For this review, take the finished solid that the model builds, in its own axes (mm). A direction names the side the tool comes from. Coordinates: 2 decimals unless noted, no trailing zeros. Loops run counter-clockwise (first coordinate to the right, second up) from the corner with the lowest first, then second, coordinate; pieces in that order, holes last. Notation, with made-up numbers: (-4.75, 32) - (32.25, 32) arc R17 cw to (32.25, 41) - close; hole circle Ø4 at (59, -7). An arc over 180 degrees is marked (long way). Use one line per item in the form item = value. Start each with the question number.
1. Machinability: for faces 1 (the face through (21, -87, 2)), 2 (the face through (27.5, -95, 2)), 3 (the face through (52.25, -102, 2)), 4 (the face through (-65, -1, 2)), which of the approach directions +Z, -Z, +X, -X, +Y, -Y give a long, thin tool a straight path to every point of the face, cutting with its end or side? Answer none if there is none.
2. To check wall thickness, follow probe 1 along Y at (x, z) = (28, 4); probe 2 along Y at (x, z) = (20.5, 2.55); probe 3 along Y at (x, z) = (-25, 2.1). State the ranges of each line that lie inside material, in increasing order.
3. Draft analysis for pull direction Y (two halves, no side actions). For faces 5 (the face through (-59, -100, 2)), 6 (the face through (29, -86, 2)), 7 (the face through (-27.5, -79, 2)), state which applies: +Y half, -Y half, draft (parallel to the pull), parting line (faces both ways), or undercut.
4. For pin 1 Ø2 at (x, z) = (-31, 1) entering from -Y; pin 2 Ø2 at (y, z) = (-102, 2) entering from -X, all flat-tipped, find the tip position at first contact; note any pin that passes through.
5. Add section A-A on x = 17.5. Give the boundary of the cut face in (y, z).
```python
from build123d import *

# Parameters (mm, degrees)
SKETCH1_W           = 130
SKETCH1_H           = 200
BOSS_EXTRUDE1_DEPTH = 4.5
CUT_EXTRUDE1_DEPTH  = 120.353466644
SKETCH3_W           = 12
SKETCH3_H           = 4.5
BOSS_EXTRUDE2_DEPTH = 4.5


with BuildPart() as part:
    # Sketch1 → Boss-Extrude1 (new body)
    with BuildSketch(Plane.XY):
        Rectangle(SKETCH1_W, SKETCH1_H)
    extrude(amount=BOSS_EXTRUDE1_DEPTH)

    # Sketch2 → Cut-Extrude1 (cut, through all)
    with BuildSketch(Plane.XY.offset(4.5)):
        Polygon((-27.5, -90), (-27.5, -100), (-22.5, -100), (-22.5, -90), (-21, -90), (-21, -83), (-22.5, -83), (-22.5, -75), (-27.5, -75), (-27.5, -83), (-29, -83), (-29, -90), align=None)
    cut_extrude1 = extrude(amount=-CUT_EXTRUDE1_DEPTH, mode=Mode.SUBTRACT)

    # Mirror1: Cut-Extrude1 across plane
    add(cut_extrude1.mirror(Plane(origin=(0, 0, 0), x_dir=(0, 0, 1), z_dir=(1, 0, 0))), mode=Mode.SUBTRACT)

    # Sketch3 → Boss-Extrude2 (add)
    with BuildSketch(Plane.XY.offset(4.5)):
        with Locations((-46.25, -102.25)):
            Rectangle(SKETCH3_W, SKETCH3_H)
        with Locations((46.25, -102.25)):
            Rectangle(SKETCH3_W, SKETCH3_H)
    extrude(amount=-BOSS_EXTRUDE2_DEPTH)


solid = part.part
```
Conclusion:
q1.face_1 = +Z, -Z
q1.face_2 = +Z, -Z, -Y
q1.face_3 = +Z, -Z, +X, -Y
q1.face_4 = +Z, -Z, -X, +Y, -Y
q2.probe_1 = -100 to -90, -83 to 100
q2.probe_2 = -100 to 100
q2.probe_3 = -75 to 100
q3.face_5 = -Y half
q3.face_6 = undercut
q3.face_7 = draft
q4.pin_1 = -100
q4.pin_2 = -52.25
q5.outline = (-100, 0) - (100, 0) - (100, 4.5) - (-100, 4.5) - close
